```python
from build123d import *

# Parameters (mm, degrees)
F2_R     = 6
F4_DEPTH = 88


with BuildPart() as f1:
    # F0 (on Front) → F1 (revolve)
    with BuildSketch(Plane.XZ):
        Polygon((-44, 140), (-44, 0), (44, 0), (44, 140), (15.6125054301, 140), (30, 133), (-30, 133), (-15.6125054301, 140), align=None)
    revolve(axis=Axis((0, 0, 0), (1, 0, 0)))

    # F2
    f2_edges = [f1.edges().sort_by_distance(p)[0] for p in [
        (-44, 0, -140),
        (44, 0, -140),
    ]]
    fillet(f2_edges, radius=F2_R)

    # F3 (on face) → F4 (cut)
    with BuildSketch(Plane(origin=(-44, 0, 0), x_dir=(0, -1, 0), z_dir=(-1, 0, 0))):
        with BuildLine():
            ThreePointArc((-4, 20.6155281281), (-13.3603892159, -16.201851746), (21, 0))
            ThreePointArc((21, 0), (16.201851746, 13.3603892159), (4, 20.6155281281))
            Line((4, 20.6155281281), (4, 16))
            Line((4, 16), (-4, 16))
            Line((-4, 16), (-4, 20.6155281281))
        make_face()
        with BuildLine():
            Line((4, 16), (4, 20.6155281281))
            ThreePointArc((4, 20.6155281281), (0, 21), (-4, 20.6155281281))
            Line((-4, 20.6155281281), (-4, 16))
            Line((-4, 16), (4, 16))
        make_face()
        with BuildLine():
            ThreePointArc((-4, 20.6155281281), (0, 21), (4, 20.6155281281))
            Line((4, 20.6155281281), (4, 28))
            Line((4, 28), (-4, 28))
            Line((-4, 28), (-4, 20.6155281281))
        make_face()
    extrude(amount=-F4_DEPTH, mode=Mode.SUBTRACT)


solid = f1.part
```
Read the model definition and answer for the solid it produces. Units are mm, in the model's axes. A direction names the side the tool comes from. Give positions to 0.01 mm unless a question says otherwise; leave off trailing zeros. Order: outer loops, then holes, each group sorted by start corner. A loop starts at its lowest first (then second) coordinate and runs counter-clockwise, first axis right, second up. Notation, with made-up numbers: (-22, 2) -> (32, 2) arc R7 cw to (32, 11) -> close; hole circle Ø9 at (78.25, 87). An arc over 180 degrees is marked (long way). One line per item, written item: value. Start each with the question number.
(1) A tool of negligible diameter and unlimited length cuts with its end or side. For faces 1 (the conical face through (29.3, 130.17, -28.91)), 2 (the flat face through (-44, 28, -2)), 3 (the flat face through (-1, -4, 24)), from which of +Z, -Z, +X, -X, +Y, -Y can it reach the whole face along a straight path? Write none if from no direction.
(2) Straight lines are drawn through the part: L1, parallel to Z at x = 1, y = 0; L2, parallel to Y at x = -10, z = 0; L3, parallel to Z at x = -24, y = 0. For each, find the intervals that lie inside material, in ascending order.
(3) Flat-ended cylindrical pins translate along their axes: P1, Ø12, axis at x = -25, y = -33, coming from the -Z side; P2, Ø6, axis at x = 18.5, z = 26, coming from the +Y side; P3, Ø12, axis at x = 1.5, y = -84.5, coming from the +Z side. Find the tip coordinate at first contact, or state that the pin passes through.
(4) The part is cut by section A-A (y = 0). Determine the outline of the cut face in (x, z), and give its area (3 significant figures).
(5) For a pull along Z with two mould halves and no side action, classify faces 4 (the cylindrical face through (-26.96, 85.19, -111.1)), 5 (the flat face through (-1, 0, 28)), 6 (the flat face through (44, 28, 2)) as released by +Z, released by -Z, zero draft, split by the parting line, or undercut.
Taken from the geometry:
1. face 1: none
1. face 2: +Z, -Z, -X, +Y, -Y
1. face 3: +X, -X
2. L1: -133 to -21, 28 to 133
2. L2: -133 to -21, 21 to 133
2. L3: -140 to -135.92, -133 to -21, 28 to 133, 135.92 to 140
3. P1: z = -137.37
3. P2: y = 138.1
3. P3: z = 107.36
4. outline: (-44, -134) arc R6 ccw to (-38, -140) -> (-15.61, -140) -> (-30, -133) -> (30, -133) -> (15.61, -140) -> (38, -140) arc R6 ccw to (44, -134) -> (44, -21) -> (-44, -21) -> close; (-44, 28) -> (44, 28) -> (44, 134) arc R6 ccw to (38, 140) -> (15.61, 140) -> (30, 133) -> (-30, 133) -> (-15.61, 140) -> (-38, 140) arc R6 ccw to (-44, 134) -> close
4. area: 19,700 mm^2
5. face 4: split by the parting line
5. face 5: undercut
5. face 6: zero draft
